Autodesk Inventor part; units mm, degrees
ref_plane "YZ Plane" through (0, 0, 0) normal (1, 0, 0) x (0, 1, 0)
ref_plane "XZ Plane" through (0, 0, 0) normal (0, 1, 0) x (-1, 0, 0)
ref_plane "XY Plane" through (0, 0, 0) normal (0, 0, 1) x (1, 0, 0)
sketch "main" plane through (0, 0, 0) normal (0, 0, 1) x (1, 0, 0)
  circle A0 centre (44.5304, -90.8931) radius 2.1844
  circle A1 centre (57.2304, -90.8931) radius 2.1844
  arc A2 (57.4426, -97.2395) -> (57.0183, -84.5466) centre (57.2304, -90.8931) ccw
  line L0 (57.0183, -84.5466) -> (52.7487, -84.5466)
  arc A3 (-82.6932, -36.7784) -> (52.7487, -84.5466) centre (52.7487, 131.3534) ccw
  line L1 (57.4426, -97.2395) -> (-37.5462, -97.2395)
  line L2 (-47.9494, -91.8239) -> (-84.9895, -38.9252)
  arc A4 (-82.6932, -36.7784) -> (-84.9895, -38.9252) centre (-83.6891, -38.0147) ccw
  arc A5 (-47.9494, -91.8239) -> (-37.5462, -97.2395) centre (-37.5462, -84.5395) ccw
  circle A6 centre (31.8304, -90.8931) radius 2.1844
  point P0 (7.1274, -71.1865)
  point P1 (-92.1475, -28.7025)
  point P2 (-44.1574, -97.2395)
  dimension "d1" = 12.7
  dimension "d2" = 101.6
  dimension "d3" = 1.5875
  dimension "d4" = 12.7
  dimension "d7" = 64.5774
  dimension "d10" = 12.7
  dimension "d15" = 125
  dimension "d16" = 12.7
  dimension "d17" = 215.9
sketch "Sketch1" plane through (0, 0, 0) normal (1, 0, 0) x (0, 1, 0)
  arc A0 (-39.5025, -3.0335) -> (-42.7248, -2.0551) centre (-41.6029, -4.1554) ccw
  line L0 (-42.7248, -2.0551) -> (-52.3306, -7.186)
  line L1 (-39.5025, -3.0335) -> (-35.7298, -10.0964)
  circle A1 centre (-122.5435, 34.4996) radius 2.0955
  circle A2 centre (-12.7, 0) radius 2.1844
  circle A3 centre (0, 0) radius 2.1844
  arc A4 (0.2122, -6.3465) -> (-0.2122, 6.3465) centre (0, 0) ccw
  line L2 (-0.2122, 6.3465) -> (-4.4817, 6.3465)
  arc A5 (-139.9236, 54.1147) -> (-4.4817, 6.3465) centre (-4.4817, 222.2465) ccw
  line L3 (0.2122, -6.3465) -> (-94.7766, -6.3465)
  line L4 (-105.1799, -0.9309) -> (-142.2199, 51.9678)
  arc A6 (-139.9236, 54.1147) -> (-142.2199, 51.9678) centre (-140.9195, 52.8784) ccw
  arc A7 (-105.1799, -0.9309) -> (-94.7766, -6.3465) centre (-94.7766, 6.3535) ccw
  circle A8 centre (-25.4, 0) radius 2.1844
  point P0 (-50.7588, -6.3465)
  point P1 (-37.7329, -6.3465)
extrude "Extrusion1" add sketch "Sketch1" along normal blind 1.5875 contours A0 L0 L3 A7 L4 A6 A5 L2 A4 L1
properties part number "Ramp" material "Acetal Resin, White"
Build history of the part. All positions in model axes, mm. Round coordinates to 2 decimals unless told otherwise and drop trailing zeros. Write each loop counter-clockwise with the first axis right and the second up, starting at its lowest first coordinate (ties: lowest second). Pieces come first, ordered by that corner, then holes. Notation, with made-up numbers: (11, -39) -> (40, -39) arc R15 cw to (40, -14) -> close; hole circle Ø11 at (-1.75, -34.75). An arc over 180 degrees is marked (long way). Put each result on its own line as item: value.
Item 1: Slice it at A-A, the plane y = -12.7. Give the cut face in (x, z), plus the area to 3 significant figures.
Here are the results:
outline: (0, -6.35) -> (1.59, -6.35) -> (1.59, -2.18) -> (0, -2.18) -> close; (0, 2.18) -> (1.59, 2.18) -> (1.59, 6.5) -> (0, 6.5) -> close
area: 13.5 mm^2
Item 2: Slice it at C-C, the plane y = -33. Give the cut face in (x, z), plus the area to 3 significant figures.
Here are the results:
outline: (0, -6.35) -> (1.59, -6.35) -> (1.59, 8.24) -> (0, 8.24) -> close
area: 23.2 mm^2
Item 3: Slice it at D-D, the plane z = 20.5. Give the cut face in (x, y), plus the area to 3 significant figures.
Here are the results:
outline: (0, -120.19) -> (1.59, -120.19) -> (1.59, -81.37) -> (0, -81.37) -> close
area: 61.6 mm^2
Item 4: Wall check: probe 1 along Z at (x, y) = (0.85, 0); probe 2 along Z at (x, y) = (1.2, -25.4); probe 3 along Z at (x, y) = (1, -116.5). Give the ranges that are in metal, low to high. Write a range as from..to.
Here are the results:
probe 1: z = -6.35..-2.18, 2.18..6.35
probe 2: z = -6.35..-2.18, 2.18..7.36
probe 3: z = 15.24..37.68
Item 5: Two-plate mould, pull along Y, no slides. Class faces 1 (the face through (0.783, -46.686, -4.171)), 2 (the face through (1.588, -74, 13)), 3 (the face through (0.783, -142.027, 54.016)): pulls with the +Y half, pulls with the -Y half, needs draft (parallel to the pull), parting line crosses it, or undercut.
Here are the results:
face 1: undercut
face 2: needs draft
face 3: parting line crosses it
Item 6: Slice it at B-B, the plane x = 1.3. Give the cut face in (y, z).
Here are the results:
outline: (-142.22, 51.97) -> (-105.18, -0.93) arc R12.7 ccw to (-94.78, -6.35) -> (-50.76, -6.35) -> (-42.72, -2.06) arc R2.38 cw to (-39.5, -3.03) -> (-37.73, -6.35) -> (0.21, -6.35) arc R6.35 ccw to (-0.21, 6.35) -> (-4.48, 6.35) arc R215.9 cw to (-139.92, 54.11) arc R1.59 ccw to start; hole circle Ø4.19 at (-122.54, 34.5); hole circle Ø4.37 at (-25.4, 0); hole circle Ø4.37 at (-12.7, 0); hole circle Ø4.37 at (0, 0)
Item 7: Flat gauge pin, fed straight in: P1, Ø2.5, axis at y = -12.7, z = 0, coming from the -X side. Where does the tip first touch, or does it go through?
Here are the results:
P1: passes through
